```python
from build123d import *

# Parameters (mm, degrees)
SKETCH_1_W          = 37
SKETCH_1_H          = 10
EXTRUDE_1_DEPTH     = 4.5
SKETCH_4_W          = 13.4
SKETCH_4_H          = 10
EXTRUDE_2_DEPTH     = 6
SKETCH_5_W          = 10.2
SKETCH_5_H          = 10
CUT_EXTRUDE_4_DEPTH = 0.2
SKETCH_6_W          = 37
SKETCH_6_H          = 10
EXTRUDE_3_DEPTH     = 2
SKETCH_2_R          = 2.25
CUT_EXTRUDE_1_DEPTH = 23.880122377
SKETCH_3_R          = 4.5
CUT_EXTRUDE_3_DEPTH = 4
SKETCH_7_W          = 9
SKETCH_7_H          = 9
CUT_EXTRUDE_5_DEPTH = 1
CHAMFER_1_SIZE      = 3
SKETCH_8_W          = 10.6
SKETCH_8_H          = 6.6
CUT_EXTRUDE_6_DEPTH = 25.464259645


with BuildPart() as part:
    # 스케치1 → 보스-돌출1 (new body)
    with BuildSketch(Plane.XY):
        Rectangle(SKETCH_1_W, SKETCH_1_H)
    extrude(amount=EXTRUDE_1_DEPTH)

    # 스케치4 → 보스-돌출2 (add)
    with BuildSketch(Plane.XY.offset(4.5)):
        with Locations((-11.8, 0)):
            Rectangle(SKETCH_4_W, SKETCH_4_H)
        with Locations((11.8, 0)):
            Rectangle(SKETCH_4_W, SKETCH_4_H)
    extrude(amount=EXTRUDE_2_DEPTH)

    # 스케치5 → 컷-돌출4 (cut)
    with BuildSketch(Plane.XY.offset(4.5)):
        Rectangle(SKETCH_5_W, SKETCH_5_H)
    extrude(amount=-CUT_EXTRUDE_4_DEPTH, mode=Mode.SUBTRACT)

    # 스케치6 → 보스-돌출3 (add)
    with BuildSketch(Plane.XY.offset(10.5)):
        Rectangle(SKETCH_6_W, SKETCH_6_H)
    extrude(amount=EXTRUDE_3_DEPTH)

    # 스케치2 → 컷-돌출1 (cut, through all)
    with BuildSketch(Plane.XY):
        with Locations(Location((0, 0, 0), (0, 0, 180))):
            Circle(SKETCH_2_R)
    extrude(amount=CUT_EXTRUDE_1_DEPTH, mode=Mode.SUBTRACT)

    # 스케치3 → 컷-돌출3 (cut)
    with BuildSketch(Plane(origin=(0, 0, 0), x_dir=(-1, 0, 0), z_dir=(0, 0, -1))):
        Circle(SKETCH_3_R)
    extrude(amount=-CUT_EXTRUDE_3_DEPTH, mode=Mode.SUBTRACT)

    # 스케치7 → 컷-돌출5 (cut)
    with BuildSketch(Plane.XY.offset(12.5)):
        Rectangle(SKETCH_7_W, SKETCH_7_H)
    extrude(amount=-CUT_EXTRUDE_5_DEPTH, mode=Mode.SUBTRACT)

    # 모따기1
    # the kernel refuses this chamfer: 3 mm, written as the material it takes off along each edge
    with BuildSketch(Plane(origin=(-26.215048964, 5, 0), x_dir=(0, 0.02749587661058649, 0.9996219169112968), z_dir=(1, 0, 0)), Plane(origin=(26.215048964, 5, 12.5), x_dir=(0, 0.027495876610586494, -0.9996219169112968), z_dir=(-1, 0, 0))) as chamfer_1_piece_1:
        Polygon((CHAMFER_1_SIZE * 0.999621916911, CHAMFER_1_SIZE * 0.0274958766106), (-CHAMFER_1_SIZE * 0.0274958766106, CHAMFER_1_SIZE * 0.999621916911), (0, 0), align=None)
    extrude(amount=52.430097928, mode=Mode.SUBTRACT)
    with BuildSketch(Plane(origin=(18.5, 5, 20.215048964), x_dir=(-0.9996219169112969, 0.027495876610586497, 0), z_dir=(0, 0, -1)), Plane(origin=(-18.5, 5, -7.715048964), x_dir=(0.9996219169112969, 0.027495876610586497, 0), z_dir=(0, 0, 1))) as chamfer_1_piece_2:
        Polygon((CHAMFER_1_SIZE * 0.999621916911, -CHAMFER_1_SIZE * 0.0274958766106), (-CHAMFER_1_SIZE * 0.0274958766106, -CHAMFER_1_SIZE * 0.999621916911), (0, 0), align=None)
    extrude(amount=27.930097928, mode=Mode.SUBTRACT)

    # 스케치8 → 컷-돌출6 (cut, through all)
    with BuildSketch(Plane(origin=(0, 5, 0), x_dir=(1, 0, 0), z_dir=(0, 1, 0))):
        with Locations((0, -7.4)):
            Rectangle(SKETCH_8_W, SKETCH_8_H)
    extrude(amount=-CUT_EXTRUDE_6_DEPTH, mode=Mode.SUBTRACT)


solid = part.part
```
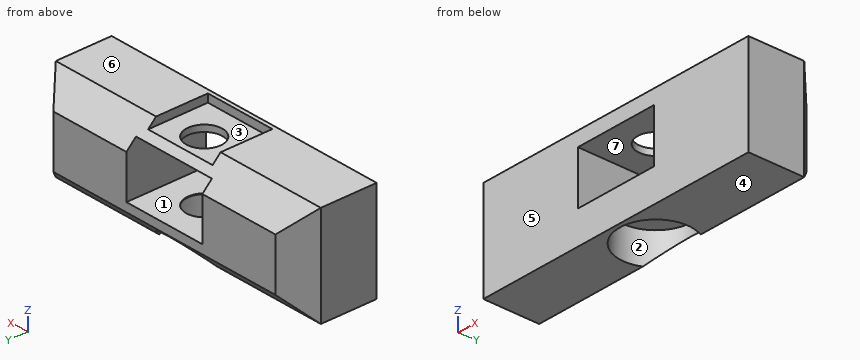
Work out the finished part from the listing and answer in its coordinate system (mm). Face numbers are marked on the shaded views. A direction names the side the tool comes from. Give positions to 0.01 mm unless a question says otherwise; leave off trailing zeros. Loops run counter-clockwise (first coordinate to the right, second up) from the corner with the lowest first, then second, coordinate; pieces in that order, holes last. Notation, with made-up numbers: M 60,76 L 108,76 A20 cw 108,108 Z; hole C 64.5,11 d7. An arc over 180 degrees is marked long. One line per item, written item: value. Start each with the question number.
1. Which of the six approach directions +Z, -Z, +X, -X, +Y, -Y give full straight-line access (tool end or side, diameter ignored) to the marked faces 1, 2, 3 and 4?
2. Find section B-B (z = 7.5). Give the vertices of the cut face in (x, y), and give its area (3 significant figures).
3. Find the intervals of material crossed by probe 1 along X at (y, z) = (-1, 8.75); probe 2 along X at (y, z) = (-3.25, 2); probe 3 along Y at (x, z) = (0, 2.3), in increasing order.
4. Find section C-C (x = 0). Give the vertices of the cut face in (y, z).
5. Find section D-D (y = -4). Give the vertices of the cut face in (x, z), and give its area (3 significant figures).
6. Find section A-A (y = 0). Give the vertices of the cut face in (x, z).
7. Each of these flat-tipped pins is pushed along its axis until it touches: P1, Ø5, axis at y = 3.5, z = 4, coming from the -X side; P2, Ø5, axis at x = 0, y = 0, coming from the +Z side; P3, Ø1.1, axis at x = -1.5, z = 12, coming from the +Y side; P4, Ø2.5, axis at x = -2, y = -1, coming from the -Z side. Where does it stop, or does it pass through?
8. Determine the mould class of the marked faces 5, 6 and 7 for opening direction Z: released by +Z, released by -Z, zero draft, split by the parting line, or undercut.
Reported:
1. face 1: +Y, -Y
1. face 2: -Z
1. face 3: +Z, +Y
1. face 4: -Z, +X, -X, +Y, -Y
2. outline: M -18.5,-5 L -5.3,-5 L -5.3,5 L -15.5,5 L -18.5,2 Z; M 5.3,-5 L 18.5,-5 L 18.5,2 L 15.5,5 L 5.3,5 Z
2. area: 255 mm²
3. probe 1: x = -18.5 to -5.3, 5.3 to 18.5
3. probe 2: x = -18.5 to -3.11, 3.11 to 18.5
3. probe 3: y = -5 to -4.5
4. outline: M -5,0 L -4.5,0 L -4.5,4 L -2.25,4 L -2.25,4.1 L -5,4.1 Z; M -5,10.7 L -2.25,10.7 L -2.25,11.5 L -4.5,11.5 L -4.5,12.5 L -5,12.5 Z; M 2.25,4 L 4.5,4 L 4.5,2.5 L 5,3 L 5,4.1 L 2.25,4.1 Z; M 2.25,10.7 L 3.8,10.7 L 3,11.5 L 2.25,11.5 Z
5. outline: M -18.5,0 L -2.06,0 L -2.06,4 L 2.06,4 L 2.06,0 L 18.5,0 L 18.5,12.5 L 4.5,12.5 L 4.5,11.5 L -4.5,11.5 L -4.5,12.5 L -18.5,12.5 Z; hole M -5.3,4.1 L 5.3,4.1 L 5.3,10.7 L -5.3,10.7 Z
5. area: 367 mm²
6. outline: M -18.5,0 L -4.5,0 L -4.5,4 L -2.25,4 L -2.25,4.1 L -5.3,4.1 L -5.3,10.7 L -2.25,10.7 L -2.25,11.5 L -4.5,11.5 L -4.5,12.5 L -18.5,12.5 Z; M 2.25,4 L 4.5,4 L 4.5,0 L 18.5,0 L 18.5,12.5 L 4.5,12.5 L 4.5,11.5 L 2.25,11.5 L 2.25,10.7 L 5.3,10.7 L 5.3,4.1 L 2.25,4.1 Z
7. P1: stops at x = -18.5
7. P2: stops at z = 11.5
7. P3: stops at y = 3.05
7. P4: stops at z = 4
8. face 5: zero draft
8. face 6: released by +Z
8. face 7: undercut
